Job drawing, mm, ordinate dimensions from the low corner. One solid piece. Round coordinates to 2 decimals unless told otherwise and drop trailing zeros. Loops run counter-clockwise (first coordinate to the right, second up) from the corner with the lowest first, then second, coordinate; pieces in that order, holes last.
1) Probe line 1 (Y direction, x = 12, z = 13) (1 decimal); line 2 (Y direction, x = 7, z = 10.25) (1 decimal); line 3 (Y direction, x = 15, z = 9.75). List the from-to ranges inside material, lowest first.
2) Band-saw the part on D-D, the plane x = 12. Write the cut outline in (y, z).
3) Mould opens along Y. For the marked faces 1, 2, 3 and 4 say: +Y half, -Y half, draft (parallel to the pull), parting line (faces both ways), or undercut.
4) Band-saw the part on B-B, the plane z = 12. Write the cut outline in (x, y).
5) Band-saw the part on C-C, the plane y = 34. Write the cut outline in (x, z), then the cut area to 3 significant figures.
6) Band-saw the part on A-A, the plane x = 5. Write the cut outline in (y, z).
7) Drop flat-ended pins along their axis: P1, Ø2, axis at y = 36, z = 13.5, coming from the +X side; P2, Ø7, axis at x = 9.59, y = 32.1, coming from the +Z side; P3, Ø10, axis at x = 29, z = 8, coming from the +Y side. Give the stop position or say it passes through.
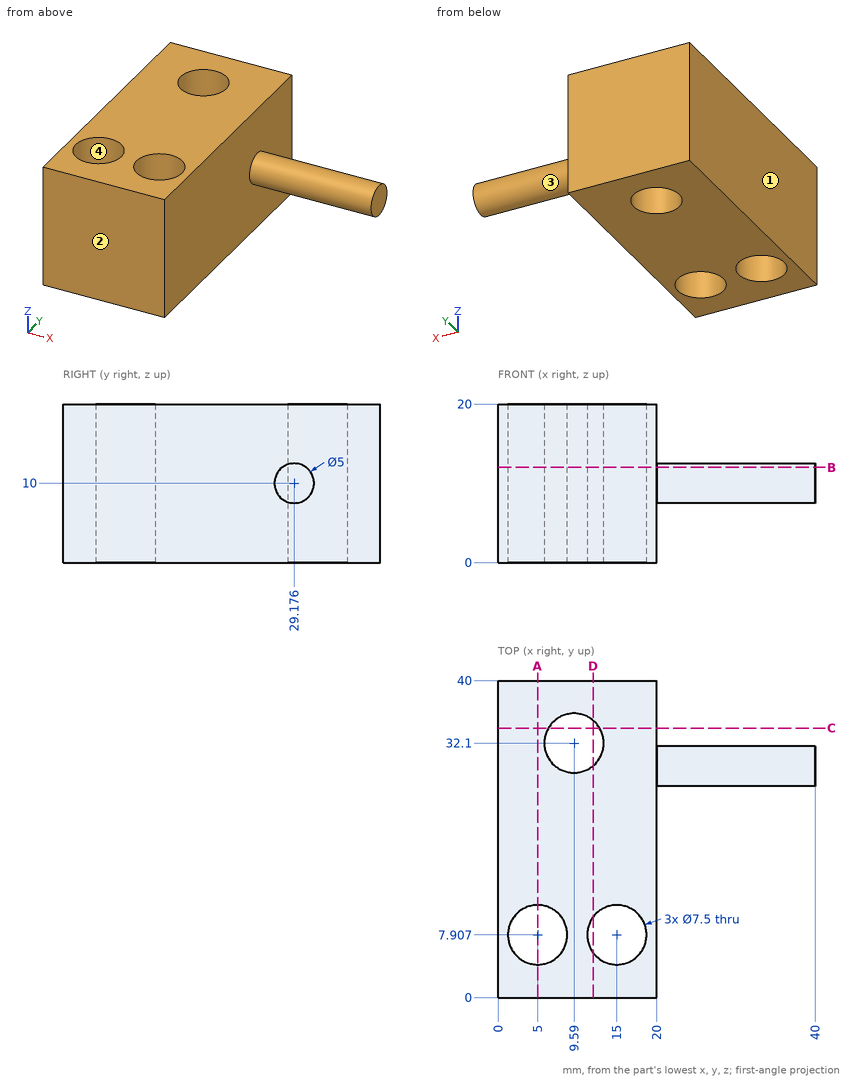
Reported:
1. line 1: y = 0 to 5.7, 10.2 to 29.2, 35 to 40
1. line 2: y = 0 to 4.7, 11.1 to 29.4, 34.8 to 40
1. line 3: y = 0 to 4.16, 11.66 to 40
2. outline: (0, 0) - (5.66, 0) - (5.66, 20) - (0, 20) - close; (10.16, 0) - (29.23, 0) - (29.23, 20) - (10.16, 20) - close; (34.97, 0) - (40, 0) - (40, 20) - (34.97, 20) - close
3. face 1: draft
3. face 2: -Y half
3. face 3: parting line
3. face 4: undercut
4. outline: (0, 0) - (20, 0) - (20, 27.68) - (40, 27.68) - (40, 30.68) - (20, 30.68) - (20, 40) - (0, 40) - close; hole circle Ø7.5 at (5, 7.91); hole circle Ø7.5 at (9.59, 32.1); hole circle Ø7.5 at (15, 7.91)
5. outline: (0, 0) - (6.36, 0) - (6.36, 20) - (0, 20) - close; (12.82, 0) - (20, 0) - (20, 20) - (12.82, 20) - close
5. area: 271 mm2
6. outline: (0, 0) - (4.16, 0) - (4.16, 20) - (0, 20) - close; (11.66, 0) - (40, 0) - (40, 20) - (11.66, 20) - close
7. P1: stops at x = 20
7. P2: passes through
7. P3: stops at y = 31.68
